```python
from build123d import *

# Parameters (mm, degrees)
EXTRUDE1_DEPTH     = 53
HOLE1_D            = 13
HOLE1_DEPTH        = 53
SKETCH5_R          = 4
CUT_EXTRUDE1_DEPTH = 4
SKETCH6_R          = 5.5
CUT_EXTRUDE2_DEPTH = 3
SKETCH7_R          = 2
CUT_EXTRUDE3_DEPTH = 33
CUT_EXTRUDE4_DEPTH = 5


with BuildPart() as part:
    # Sketch1 → Extrude1 (new body)
    with BuildSketch(Plane(origin=(0, 0, 0), x_dir=(1, 0, 0), z_dir=(0, 1, 0))):
        with BuildLine():
            Line((-48.427781283, 31), (48.427781283, 31))
            ThreePointArc((48.427781283, 31), (57.5, 0), (48.427781283, -31))
            Line((48.427781283, -31), (-48.427781283, -31))
            ThreePointArc((-48.427781283, -31), (-57.5, 0), (-48.427781283, 31))
        make_face()
    extrude(amount=EXTRUDE1_DEPTH)

    # Sketch2 → Revolve1 (revolve)
    with BuildSketch(Plane.XY, mode=Mode.PRIVATE) as revolve1_sk:
        Polygon((0, 91), (-8.25, 91), (-8.25, 75), (-18, 75), (-18, 74), (-30.95, 74), (-30.95, 53), (0, 53), align=None)
    revolve(revolve1_sk.sketch.rotate(Axis((0, 0, 0), (0, 1, 0)), 270), axis=Axis((0, 0, 0), (0, 1, 0)))  # turned: the seam where the file's is

    # Hole1
    with Locations(Plane(origin=(0, 53, 0), x_dir=(-1, 0, 0), z_dir=(0, 1, 0))):
        with Locations((45, 0), (-45, 0)):
            Hole(HOLE1_D / 2, depth=HOLE1_DEPTH)

    # Sketch5 → Cut-Extrude1 (cut)
    with BuildSketch(Plane.XZ):
        with Locations(Location((0, 0, 0), (0, 0, 270))):  # turned: the seam where the file's is
            Circle(SKETCH5_R)
    extrude(amount=-CUT_EXTRUDE1_DEPTH, mode=Mode.SUBTRACT)

    # Sketch6 → Cut-Extrude2 (cut)
    with BuildSketch(Plane.XZ):
        with Locations(Location((35, -15, 0), (0, 0, 270))):  # turned: the seam where the file's is
            Circle(SKETCH6_R)
    extrude(amount=-CUT_EXTRUDE2_DEPTH, mode=Mode.SUBTRACT)

    # Sketch7 → Cut-Extrude3 (cut)
    with BuildSketch(Plane.XZ.offset(-3)):
        with Locations(Location((35, -15, 0), (0, 0, 270))):  # turned: the seam where the file's is
            Circle(SKETCH7_R)
    extrude(amount=-CUT_EXTRUDE3_DEPTH, mode=Mode.SUBTRACT)

    # Sketch8 → Cut-Revolve1 (revolve, cut)
    with BuildSketch(Plane(origin=(0, 0, 0), x_dir=(0.920504853, 0, -0.390731128), z_dir=(0.390731128, 0, 0.920504853)), mode=Mode.PRIVATE) as cut_revolve1_sk:
        Polygon((57.5, 28), (55, 28), (55, 33.4215), (53.517364509, 34.2775), (35, 34.2775), (35, 40), (57.5, 40), align=None)
    revolve(cut_revolve1_sk.sketch.rotate(Axis((47.484793311, 40, -20.156098913), (-0.920504853, 0, 0.390731128)), 270), axis=Axis((47.484793311, 40, -20.156098913), (-0.920504853, 0, 0.390731128)), mode=Mode.SUBTRACT)  # turned: the seam where the file's is

    # Sketch9 → Revolve2 (revolve)
    with BuildSketch(Plane(origin=(0, 0, 0), x_dir=(0.920504853, 0, -0.390731128), z_dir=(0.390731128, 0, 0.920504853)), mode=Mode.PRIVATE) as revolve2_sk:
        Polygon((55, 31), (55, 34.2775), (46, 34.2775), (45, 35.2775), (45, 40), (60, 40), (60, 31), align=None)
    revolve(revolve2_sk.sketch.rotate(Axis((68.658528533, 40, -29.14381628), (-0.920504853, 0, 0.390731128)), 270), axis=Axis((68.658528533, 40, -29.14381628), (-0.920504853, 0, 0.390731128)))  # turned: the seam where the file's is

    # Sketch10 → Cut-Extrude4 (cut)
    with BuildSketch(Plane(origin=(55.230291207, 0, -23.443867709), x_dir=(-0.390731128, 0, -0.920504853), z_dir=(0.920504853, 0, -0.390731128))):
        Polygon((4.041451884, 40), (2.020725942, 43.5), (-2.020725942, 43.5), (-4.041451884, 40), (-2.020725942, 36.5), (2.020725942, 36.5), align=None)
    extrude(amount=-CUT_EXTRUDE4_DEPTH, mode=Mode.SUBTRACT)


solid = part.part
```
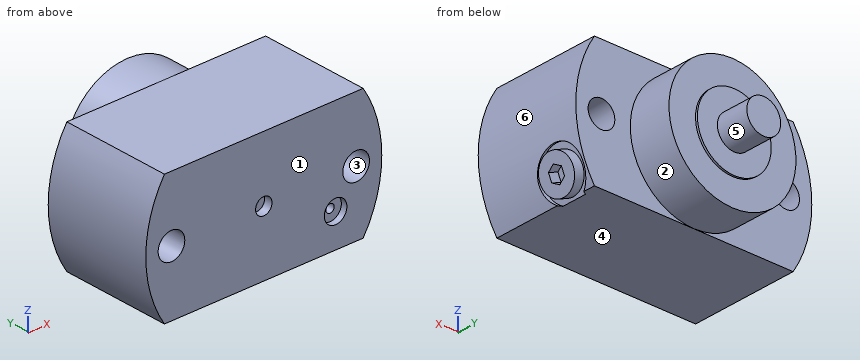
CAD build for the part. Positions are in the model's coordinates, mm. Face numbers are marked on the shaded views. A direction names the side the tool comes from. Coordinates: 2 decimals unless noted, no trailing zeros. Order: outer loops, then holes, each group sorted by start corner. A loop starts at its lowest first (then second) coordinate and runs counter-clockwise, first axis right, second up.
(1) Pin check, flat tips, straight feed: pin 1 Ø2.5 at (x, z) = (35, -15) entering from +Y; pin 2 Ø1 at (x, z) = (19, 8) entering from +Y; pin 3 Ø12 at (y, z) = (15.5, -13.5) entering from +X. Stop position of each tip, or through.
Solution:
pin 1: stops at y = 53
pin 2: stops at y = 74
pin 3: stops at x = 57.01
(2) Which spindle directions (+Z, -Z, +X, -X, +Y, -Y) get a long thin tool onto all of the face, cutting with end or side? Do the marked faces 1 and 2. Say none if no direction does.
Solution:
face 1: +Z, -Z, +X, -X, -Y
face 2: +Y
(3) Saw through at A-A, the plane x = -45. Write the cut outline in (y, z), and give its area (3 significant figures).
Solution:
outline: (0, -31) - (53, -31) - (53, -6.5) - (0, -6.5) - close; (0, 6.5) - (53, 6.5) - (53, 31) - (0, 31) - close
area: 2,600 mm2
(4) Mould opens along X. For the marked faces 3, 4, 5 and 6 say: released by +X, released by -X, zero draft, split by the parting line, or undercut.
Solution:
face 3: undercut
face 4: zero draft
face 5: split by the parting line
face 6: released by +X
(5) Saw through at D-D, the plane z = 15. Write the cut outline in (x, y).
Solution:
outline: (-55.51, 0) - (55.51, 0) - (55.51, 53) - (27.07, 53) - (27.07, 74) - (9.95, 74) - (9.95, 75) - (-9.95, 75) - (-9.95, 74) - (-27.07, 74) - (-27.07, 53) - (-55.51, 53) - close
(6) Saw through at C-C, the plane x = 0. Write the cut outline in (y, z).
Solution:
outline: (0, -31) - (53, -31) - (53, -30.95) - (74, -30.95) - (74, -18) - (75, -18) - (75, -8.25) - (91, -8.25) - (91, 8.25) - (75, 8.25) - (75, 18) - (74, 18) - (74, 30.95) - (53, 30.95) - (53, 31) - (0, 31) - (0, 4) - (4, 4) - (4, -4) - (0, -4) - close
(7) Drill centre lines: L1, parallel to Y at x = -3.5, z = 16.5; L2, parallel to Z at x = 6, y = 42; L3, parallel to Y at x = -27, z = 2.5. Where is each one in solid material? Low to high.
Solution:
L1: y = 0 to 75
L2: z = -31 to 31
L3: y = 0 to 74
(8) Saw through at B-B, the plane z = 0. Write the cut outline in (x, y), and give its area (3 significant figures).
Solution:
outline: (-57.5, 0) - (-51.5, 0) - (-51.5, 53) - (-57.5, 53) - close; (-38.5, 0) - (-4, 0) - (-4, 4) - (4, 4) - (4, 0) - (38.5, 0) - (38.5, 53) - (30.95, 53) - (30.95, 74) - (18, 74) - (18, 75) - (8.25, 75) - (8.25, 91) - (-8.25, 91) - (-8.25, 75) - (-18, 75) - (-18, 74) - (-30.95, 74) - (-30.95, 53) - (-38.5, 53) - close; (51.5, 0) - (57.5, 0) - (57.5, 53) - (51.5, 53) - close
area: 6,280 mm2
